Can you work these out from the model? Positions are in its coordinate system, mm. A direction names the side the tool comes from. Give positions to 0.01 mm unless a question says otherwise; leave off trailing zeros. Loops run counter-clockwise (first coordinate to the right, second up) from the corner with the lowest first, then second, coordinate; pieces in that order, holes last. Notation, with made-up numbers: (-9.5, 18) -> (17.5, 18) arc R15 ccw to (17.5, 26) -> close; hole circle Ø9 at (40.5, 12). An arc over 180 degrees is marked (long way). Return JSON: item names as keys, results as strings. Group by question number.
Q1. Suppose I cut it at D-D, the plane z = -9. Please give me the cut outline in (x, y), and give its area (3 significant figures).
Q2. Will these pins go through, and if not, where does the flat tip stop? pin 1 (6 mm diameter, centred on x = 15.5, z = -19, fed in from +Y); pin 2 (2 mm diameter, centred on x = 10.5, y = 34, fed in from +Z); pin 3 (1.9 mm diameter, centred on x = -0.5, z = 1.5, fed in from +Y); pin 4 (3 mm diameter, centred on y = 57.5, z = -16, fed in from +X).
Q3. Which directions (+Z, -Z, +X, -X, +Y, -Y) give clear straight access to the entire face, cutting with the end or side of a thin tool? Please do faces 1 (the cylindrical face through (-1.72, 60.35, 7.75)), 2 (the flat face through (0, 0, 0)), 3 (the cylindrical face through (-5, 5, 22.5)).
Q4. I need wall thicknesses on line 1 along X through (y, z) = (53.5, 0) (3 decimals); line 2 along Z through (x, y) = (0, 55.25) (1 decimal). Which ranges of each line are inside material? Lowest first, please. Write a range as [from, to].
```python
from build123d import *

# Parameters (mm, degrees)
SKETCH1_R           = 23.0505
BOSS_EXTRUDE1_DEPTH = 10.16
SKETCH2_R           = 24.4856
BOSS_EXTRUDE2_DEPTH = 4.064
SKETCH3_R           = 19.05
BOSS_EXTRUDE3_DEPTH = 20.066
SKETCH4_R           = 18.034
BOSS_EXTRUDE4_DEPTH = 20.32
SKETCH5_R           = 7.9375
BOSS_EXTRUDE5_DEPTH = 11.6332
SKETCH7_R           = 3.175
CUT_EXTRUDE1_DEPTH  = 17.018
CHAMFER1_SIZE       = 2.286
CHAMFER1_SIZE2      = 2.794


with BuildPart() as part:
    # Sketch1 → Boss-Extrude1 (new body)
    with BuildSketch(Plane(origin=(0, 0, 0), x_dir=(1, 0, 0), z_dir=(0, 1, 0))):
        Circle(SKETCH1_R)
    extrude(amount=BOSS_EXTRUDE1_DEPTH)

    # Sketch2 → Boss-Extrude2 (add)
    with BuildSketch(Plane(origin=(0, 10.16, 0), x_dir=(1, 0, 0), z_dir=(0, 1, 0))):
        Circle(SKETCH2_R)
    extrude(amount=BOSS_EXTRUDE2_DEPTH)

    # Sketch3 → Boss-Extrude3 (add)
    with BuildSketch(Plane(origin=(0, 14.224, 0), x_dir=(1, 0, 0), z_dir=(0, 1, 0))):
        Circle(SKETCH3_R)
    extrude(amount=BOSS_EXTRUDE3_DEPTH)

    # Sketch4 → Boss-Extrude4 (add)
    with BuildSketch(Plane(origin=(0, 34.29, 0), x_dir=(1, 0, 0), z_dir=(0, 1, 0))):
        Circle(SKETCH4_R)
    extrude(amount=BOSS_EXTRUDE4_DEPTH)

    # Sketch5 → Boss-Extrude5 (add)
    with BuildSketch(Plane(origin=(0, 54.61, 0), x_dir=(1, 0, 0), z_dir=(0, 1, 0))):
        Circle(SKETCH5_R)
    extrude(amount=BOSS_EXTRUDE5_DEPTH)

    # Sketch7 → Cut-Extrude1 (cut)
    with BuildSketch(Plane(origin=(0, 66.2432, 0), x_dir=(1, 0, 0), z_dir=(0, 1, 0))):
        Circle(SKETCH7_R)
    extrude(amount=-CUT_EXTRUDE1_DEPTH, mode=Mode.SUBTRACT)

    # Chamfer1
    chamfer1_edges = [part.edges().sort_by_distance(p)[0] for p in [
        (-3.175, 66.2432, 0),
    ]]
    chamfer1_side = [part.faces().sort_by_distance(p)[0] for p in [
        (-7.712993597, 66.2432, 0),
    ]]
    chamfer(chamfer1_edges, length=CHAMFER1_SIZE, length2=CHAMFER1_SIZE2, reference=chamfer1_side[0])


solid = part.part
```
Ans:
{
 "1": {"outline": "(-22.77, 10.16) -> (-21.22, 10.16) -> (-21.22, 0) -> (21.22, 0) -> (21.22, 10.16) -> (22.77, 10.16) -> (22.77, 14.22) -> (16.79, 14.22) -> (16.79, 34.29) -> (15.63, 34.29) -> (15.63, 54.61) -> (-15.63, 54.61) -> (-15.63, 34.29) -> (-16.79, 34.29) -> (-16.79, 14.22) -> (-22.77, 14.22) -> close", "area": "1,930 mm^2"},
 "2": {"pin 1": "stops at y = 14.22", "pin 2": "stops at z = 16.51", "pin 3": "stops at y = 49.23", "pin 4": "passes through"},
 "3": {"face 1": "+Y", "face 2": "+Z, -Z, +X, -X, -Y", "face 3": "-Y"},
 "4": {"line 1": "x = [-18.034, -3.175], [3.175, 18.034]", "line 2": "z = [-7.9, -3.2], [3.2, 7.9]"}
}
